Read the model definition and answer for the solid it produces. Units are mm, in the model's axes. A direction names the side the tool comes from. Give positions to 0.01 mm unless a question says otherwise; leave off trailing zeros. Write each loop counter-clockwise with the first axis right and the second up, starting at its lowest first coordinate (ties: lowest second). Pieces come first, ordered by that corner, then holes. Notation, with made-up numbers: (8, -21) -> (31, -21) arc R15 ccw to (31, -17) -> close; hole circle Ø10 at (42, -8). An arc over 180 degrees is marked (long way). Use a Markdown table: item, result.
from build123d import *

# Parameters (mm, degrees)
F0_W     = 500
F0_H     = 20
F4_DEPTH = 150
F1_W     = 20
F1_H     = 250
F5_DEPTH = 150
F2_W     = 20
F2_H     = 250
F6_DEPTH = 150
F3_W     = 460
F3_H     = 175
F7_DEPTH = 10


with BuildPart() as f4:
    # F0 (on Front) → F4 (new body, symmetric)
    with BuildSketch(Plane.XZ):
        Rectangle(F0_W, F0_H)
    extrude(amount=F4_DEPTH, both=True)

    # F1 (on Front) → F5 (join, symmetric)
    with BuildSketch(Plane.XZ):
        with Locations((-240, -135)):
            Rectangle(F1_W, F1_H)
    extrude(amount=F5_DEPTH, both=True)

    # F2 (on Front) → F6 (join, symmetric)
    with BuildSketch(Plane.XZ):
        with Locations((240, -135)):
            Rectangle(F2_W, F2_H)
    extrude(amount=F6_DEPTH, both=True)

    # F3 (on Front) → F7 (join, symmetric)
    with BuildSketch(Plane.XZ):
        with Locations((0, -97.5)):
            Rectangle(F3_W, F3_H)
    extrude(amount=F7_DEPTH, both=True)


solid = f4.part
Item 1: A tool of negligible diameter and unlimited length cuts with its end or side. For faces 5 (the face through (240, -2, -260)), 6 (the face through (-3, 79, -10)), 7 (the face through (-3, -2, 10)), 8 (the face through (-3, -10, -96)), 9 (the face through (-230, -35, -137)), from which of +Z, -Z, +X, -X, +Y, -Y can it reach the whole face along a straight path? Write none if from no direction.
Return value:
| item | result |
|---|---|
| face 5 | -Z, +X, -X, +Y, -Y |
| face 6 | -Z, +Y |
| face 7 | +Z, +X, -X, +Y, -Y |
| face 8 | -Z, -Y |
| face 9 | -Z |
Item 2: A cutting plane is placed at D-D (y = -72). Give the vertices of the cut face in (x, z), then the cut area to 3 significant figures.
Return value:
| item | result |
|---|---|
| outline | (-250, -260) -> (-230, -260) -> (-230, -10) -> (230, -10) -> (230, -260) -> (250, -260) -> (250, 10) -> (-250, 10) -> close |
| area | 20,000 mm^2 |
Item 3: A cutting plane is placed at B-B (x = -85). Give the vertices of the cut face in (y, z), then the cut area to 3 significant figures.
Return value:
| item | result |
|---|---|
| outline | (-150, -10) -> (-10, -10) -> (-10, -185) -> (10, -185) -> (10, -10) -> (150, -10) -> (150, 10) -> (-150, 10) -> close |
| area | 9,500 mm^2 |
Item 4: A cutting plane is placed at C-C (z = -48). Give the vertices of the cut face in (x, y), then the cut area to 3 significant figures.
Return value:
| item | result |
|---|---|
| outline | (-250, -150) -> (-230, -150) -> (-230, -10) -> (230, -10) -> (230, -150) -> (250, -150) -> (250, 150) -> (230, 150) -> (230, 10) -> (-230, 10) -> (-230, 150) -> (-250, 150) -> close |
| area | 21,200 mm^2 |
Item 5: Straight lines are drawn through the part: line 1 along X through (y, z) = (-43, -233); line 2 along Z through (x, y) = (96, 2); line 3 along Z through (x, y) = (220, -58.5). For each, find the intervals that lie inside material, in ascending order. Write a range as [from, to].
Return value:
| item | result |
|---|---|
| line 1 | [-250, -230], [230, 250] |
| line 2 | [-185, 10] |
| line 3 | [-10, 10] |
Item 6: For a pull along X with two mould halves and no side action, classify faces 1 (the face through (-3, 0, -185)), 2 (the face through (-250, -2, -127)), 3 (the face through (-20, 150, -4)), 4 (the face through (230, -35, -137)) as +X half, -X half, draft (parallel to the pull), parting line (faces both ways), or undercut.
Return value:
| item | result |
|---|---|
| face 1 | undercut |
| face 2 | -X half |
| face 3 | draft |
| face 4 | undercut |
Item 7: Each of these flat-tipped pins is pushed along its axis until it touches: P1, Ø5, axis at x = -168.5, z = -183.5, coming from the -Y side; P2, Ø6, axis at x = -171.5, z = -62, coming from the +Y side; P3, Ø4, axis at x = -1, y = -106, coming from the -Z side. Where does it stop, or does it pass through?
Return value:
| item | result |
|---|---|
| P1 | y = -10 |
| P2 | y = 10 |
| P3 | z = -10 |
Item 8: A cutting plane is placed at A-A (z = -205.5). Give the vertices of the cut face in (x, y).
Return value:
| item | result |
|---|---|
| outline | (-250, -150) -> (-230, -150) -> (-230, 150) -> (-250, 150) -> close; (230, -150) -> (250, -150) -> (250, 150) -> (230, 150) -> close |
